The listing builds one solid part. Answer for the finished solid, in the listing's coordinates (mm). A direction names the side the tool comes from. Give positions to 0.01 mm unless a question says otherwise; leave off trailing zeros. Write each loop counter-clockwise with the first axis right and the second up, starting at its lowest first coordinate (ties: lowest second). Pieces come first, ordered by that corner, then holes. Notation, with made-up numbers: M 10.5,78.5 L 24.5,78.5 A34 ccw 24.5,114.5 Z; hole C 6.25,44.25 d5. An arc over 180 degrees is marked long. Return JSON: item names as keys, results as strings.
from build123d import *

# Parameters (mm, degrees)
SKETCH1_W           = 70
SKETCH1_H           = 48
SKETCH1_R           = 0.5
SKETCH1_R_2         = 1.4
BOSS_EXTRUDE1_DEPTH = 1
SKETCH2_W           = 62.5
SKETCH2_H           = 40
BOSS_EXTRUDE2_DEPTH = 3.3
SKETCH3_W           = 60
SKETCH3_H           = 43
BOSS_EXTRUDE3_DEPTH = 2


with BuildPart() as part:
    # Sketch1 → Boss-Extrude1 (new body)
    with BuildSketch(Plane(origin=(0, 0, 0), x_dir=(1, 0, 0), z_dir=(0, 1, 0))):
        with Locations((-35, 24)):
            Rectangle(SKETCH1_W, SKETCH1_H)
        with Locations(Location((-68.2, 20.4, 0), (0, 0, 270))):
            Circle(SKETCH1_R, mode=Mode.SUBTRACT)
        with Locations(Location((-68.2, 22.8, 0), (0, 0, 270))):
            Circle(SKETCH1_R, mode=Mode.SUBTRACT)
        with Locations(Location((-68.2, 25.2, 0), (0, 0, 270))):
            Circle(SKETCH1_R, mode=Mode.SUBTRACT)
        with Locations(Location((-68.2, 27.6, 0), (0, 0, 270))):
            Circle(SKETCH1_R, mode=Mode.SUBTRACT)
        with Locations(Location((-31.4, 45.2, 0), (0, 0, 270))):
            Circle(SKETCH1_R, mode=Mode.SUBTRACT)
        with Locations(Location((-33.8, 45.2, 0), (0, 0, 270))):
            Circle(SKETCH1_R, mode=Mode.SUBTRACT)
        with Locations(Location((-36.2, 45.2, 0), (0, 0, 270))):
            Circle(SKETCH1_R, mode=Mode.SUBTRACT)
        with Locations(Location((-38.6, 45.2, 0), (0, 0, 270))):
            Circle(SKETCH1_R, mode=Mode.SUBTRACT)
        with Locations(Location((-67.8, 45.8, 0), (0, 0, 270))):
            Circle(SKETCH1_R_2, mode=Mode.SUBTRACT)
        with Locations(Location((-67.8, 2.2, 0), (0, 0, 270))):
            Circle(SKETCH1_R_2, mode=Mode.SUBTRACT)
        with Locations(Location((-2.2, 2.2, 0), (0, 0, 270))):
            Circle(SKETCH1_R_2, mode=Mode.SUBTRACT)
        with Locations(Location((-2.2, 45.8, 0), (0, 0, 270))):
            Circle(SKETCH1_R_2, mode=Mode.SUBTRACT)
    extrude(amount=BOSS_EXTRUDE1_DEPTH)

    # Sketch2 → Boss-Extrude2 (add)
    with BuildSketch(Plane(origin=(0, 1, 0), x_dir=(1, 0, 0), z_dir=(0, 1, 0))):
        with Locations((-35, 23.5)):
            Rectangle(SKETCH2_W, SKETCH2_H)
    extrude(amount=BOSS_EXTRUDE2_DEPTH)

    # Sketch3 → Boss-Extrude3 (add)
    with BuildSketch(Plane.XZ):
        with Locations((-35, -21.5)):
            Rectangle(SKETCH3_W, SKETCH3_H)
    extrude(amount=BOSS_EXTRUDE3_DEPTH)


solid = part.part
Item 1: A cutting plane is placed at C-C, the plane x = -21. Write down the section's boundary in (y, z).
Geometry results:
{"outline": "M -2,-43 L 0,-43 L 0,-48 L 1,-48 L 1,-43.5 L 4.3,-43.5 L 4.3,-3.5 L 1,-3.5 L 1,0 L -2,0 Z"}
Item 2: Determine the mould class of faces 6 (the cylindrical face through (-66.41, 0.49, -2.38)), 7 (the flat face through (-35, -1, 0)), 8 (the flat face through (-35, 3, -43.5)) for opening direction Z: +Z half, -Z half, draft (parallel to the pull), parting line (faces both ways), or undercut.
Geometry results:
{"face 6": "undercut", "face 7": "+Z half", "face 8": "-Z half"}
Item 3: A cutting plane is placed at B-B, the plane x = -2.2. Write down the section's boundary in (y, z).
Geometry results:
{"outline": "M 0,-48 L 1,-48 L 1,-47.2 L 0,-47.2 Z; M 0,-44.4 L 1,-44.4 L 1,-3.6 L 0,-3.6 Z; M 0,-0.8 L 1,-0.8 L 1,0 L 0,0 Z"}
Item 4: A cutting plane is placed at D-D, the plane z = -33. Write down the section's boundary in (x, y), plus the area to 3 significant figures.
Geometry results:
{"outline": "M -70,0 L -65,0 L -65,-2 L -5,-2 L -5,0 L 0,0 L 0,1 L -3.75,1 L -3.75,4.3 L -66.25,4.3 L -66.25,1 L -70,1 Z", "area": "396 mm2"}
Item 5: Which of the six approach directions +Z, -Z, +X, -X, +Y, -Y give full straight-line access (tool end or side, diameter ignored) to faces 1 (the flat face through (-5, -1, -22)), 2 (the flat face through (-35, -1, -43)), 3 (the flat face through (-65, -1, -22)), 4 (the flat face through (-3.75, 3, -23)), 5 (the flat face through (-66.25, 3, -23))?
Geometry results:
{"face 1": "+Z, -Z, +X, -Y", "face 2": "-Z, +X, -X, -Y", "face 3": "+Z, -Z, -X, -Y", "face 4": "+Z, -Z, +X, +Y", "face 5": "+Z, -Z, -X, +Y"}
Item 6: A cutting plane is placed at A-A, the plane z = -2.2. Write down the section's boundary in (x, y).
Geometry results:
{"outline": "M -70,0 L -69.2,0 L -69.2,1 L -70,1 Z; M -66.4,0 L -65,0 L -65,-2 L -5,-2 L -5,0 L -3.6,0 L -3.6,1 L -66.4,1 Z; M -0.8,0 L 0,0 L 0,1 L -0.8,1 Z"}
Item 7: Given pin 1 Ø2.5 at (y, z) = (2.5, -27) entering from +X; pin 2 Ø2 at (y, z) = (-1.5, -18.5) entering from +X; pin 3 Ø3 at (x, z) = (-2.2, -45.8) entering from -Y, each flat-ended and moving along its own axis, determine where each tip first touches the part or whether it passes through.
Geometry results:
{"pin 1": "stops at x = -3.75", "pin 2": "stops at x = -5", "pin 3": "stops at y = 0"}
Item 8: Find the intervals of material crossed by line 1 (X direction, y = 0.7, z = -2.2); line 2 (Z direction, x = -38.6, y = 0.45); line 3 (X direction, y = 0.4, z = -20.4), in increasing order.
Geometry results:
{"line 1": "x = -70 to -69.2, -66.4 to -3.6, -0.8 to 0", "line 2": "z = -48 to -45.7, -44.7 to 0", "line 3": "x = -70 to -68.7, -67.7 to 0"}
